Design review of the part shown in the three views and the two pictorial views. Dimensions are in mm from the part's minimum x, y and z. A direction names the side the tool comes from. Round coordinates to 2 decimals unless told otherwise and drop trailing zeros. Write each loop counter-clockwise with the first axis right and the second up, starting at its lowest first coordinate (ties: lowest second). Pieces come first, ordered by that corner, then holes. Notation, with made-up numbers: (66.5, 9) -> (75.5, 9) arc R14 cw to (75.5, 23) -> close; hole circle Ø5 at (-2, 56.25). An arc over 180 degrees is marked (long way). Return JSON: item names as keys, results as strings. Group by question number.
1. Clearance check with flat-ended pins moving along their axes: P1, Ø0.8, axis at x = 6.5, z = 1, coming from the -Y side; P2, Ø1, axis at x = 13.5, z = 4.5, coming from the +Y side; P3, Ø1.6, axis at y = 39, z = 0.5, coming from the -X side; P4, Ø2, axis at x = 2.5, z = 7, coming from the +Y side. State where each tip first meets the part, or that it passes through.
2. For line 1 along Y through (x, z) = (11.25, 0.85); line 2 along Y through (x, z) = (10, 4.5); line 3 along Y through (x, z) = (8, 1.25), list the stretches that pass through material, from the lowest coordinate up. Write a range as from..to.
3. Tool access review of the marked faces 1, 2, 3, 4 and 5: name each direction out of +Z, -Z, +X, -X, +Y, -Y from which nothing blocks a thin tool from reaching the whole face with its end or side.
4. Take a section at C-C, the plane x = 6.75. Write out the cut boundary in (y, z).
5. Take a section at D-D, the plane z = 5.5. Write out the cut boundary in (x, y), then the cut area to 3 significant figures.
6. Take a section at B-B, the plane y = 38. Write out the cut boundary in (x, z).
7. Take a section at A-A, the plane x = 11.25. Write out the cut boundary in (y, z).
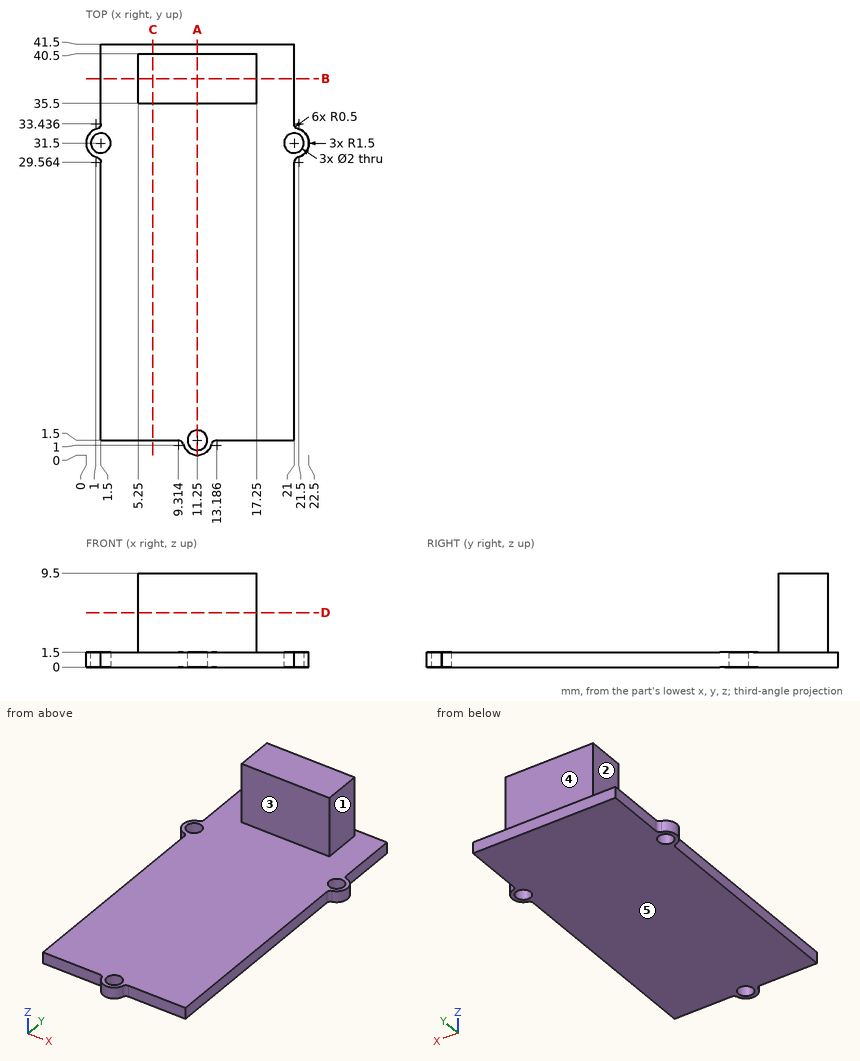
Output:
{
 "1": {"P1": "stops at y = 1.5", "P2": "stops at y = 40.5", "P3": "stops at x = 1.5", "P4": "passes through"},
 "2": {"line 1": "y = 0..0.5, 2.5..41.5", "line 2": "y = 35.5..40.5", "line 3": "y = 1.5..41.5"},
 "3": {"face 1": "+Z, +X, +Y, -Y", "face 2": "+Z, -X, +Y, -Y", "face 3": "+Z, +X, -X, -Y", "face 4": "+Z, +X, -X, +Y", "face 5": "-Z, +X, -X, +Y, -Y"},
 "4": {"outline": "(1.5, 0) -> (41.5, 0) -> (41.5, 1.5) -> (40.5, 1.5) -> (40.5, 9.5) -> (35.5, 9.5) -> (35.5, 1.5) -> (1.5, 1.5) -> close"},
 "5": {"outline": "(5.25, 35.5) -> (17.25, 35.5) -> (17.25, 40.5) -> (5.25, 40.5) -> close", "area": "60.0 mm^2"},
 "6": {"outline": "(1.5, 0) -> (21, 0) -> (21, 1.5) -> (17.25, 1.5) -> (17.25, 9.5) -> (5.25, 9.5) -> (5.25, 1.5) -> (1.5, 1.5) -> close"},
 "7": {"outline": "(0, 0) -> (0.5, 0) -> (0.5, 1.5) -> (0, 1.5) -> close; (2.5, 0) -> (41.5, 0) -> (41.5, 1.5) -> (40.5, 1.5) -> (40.5, 9.5) -> (35.5, 9.5) -> (35.5, 1.5) -> (2.5, 1.5) -> close"}
}
